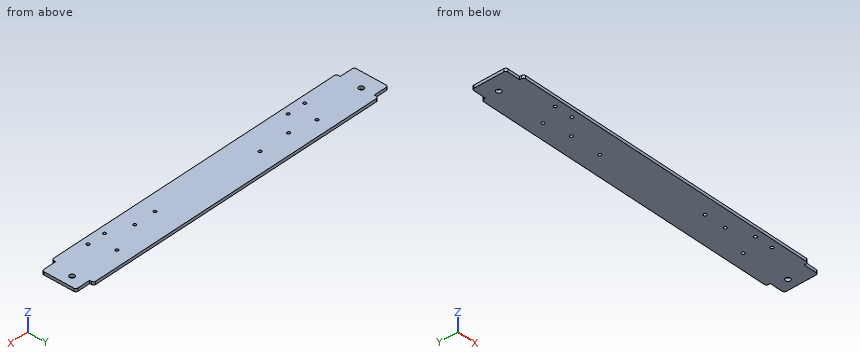
```python
from build123d import *

# Parameters (mm, degrees)
CROQUIS1_W                                 = 340
CROQUIS1_H                                 = 42
CROQUIS1_R                                 = 1.5
CROQUIS1_R_2                               = 2.5
SALIENTE_EXTRUIR1_DEPTH                    = 3
CROQUIS2_W                                 = 15
CROQUIS2_H                                 = 4
CORTAR_EXTRUIR2_DEPTH                      = 172.31841699
SIMETR_A4_AT_THE_SECOND_PLANE_COPY_1_SKE_W = 15
SIMETR_A4_AT_THE_SECOND_PLANE_COPY_1_SKE_H = 4
SIMETR_A4_AT_THE_SECOND_PLANE_COPY_1_DEPTH = 172.31841699
REDONDEO1_R                                = 2


with BuildPart() as part:
    # Croquis1 → Saliente-Extruir1 (new body)
    with BuildSketch(Plane.XY):
        Rectangle(CROQUIS1_W, CROQUIS1_H)
        with Locations((-47, 2)):
            Circle(CROQUIS1_R, mode=Mode.SUBTRACT)
        with Locations((-78, 2)):
            Circle(CROQUIS1_R, mode=Mode.SUBTRACT)
        with Locations((-104, 6.5)):
            Circle(CROQUIS1_R, mode=Mode.SUBTRACT)
        with Locations((-113, -14)):
            Circle(CROQUIS1_R, mode=Mode.SUBTRACT)
        with Locations((-95, -14)):
            Circle(CROQUIS1_R, mode=Mode.SUBTRACT)
        with Locations((-155, 4)):
            Circle(CROQUIS1_R_2, mode=Mode.SUBTRACT)
        with Locations((160, 4)):
            Circle(CROQUIS1_R_2, mode=Mode.SUBTRACT)
        with Locations((114, 6.5)):
            Circle(CROQUIS1_R, mode=Mode.SUBTRACT)
        with Locations((105, -14)):
            Circle(CROQUIS1_R, mode=Mode.SUBTRACT)
        with Locations((123, -14)):
            Circle(CROQUIS1_R, mode=Mode.SUBTRACT)
        with Locations((82, -5)):
            Circle(CROQUIS1_R, mode=Mode.SUBTRACT)
        with Locations((60, -5)):
            Circle(CROQUIS1_R, mode=Mode.SUBTRACT)
    extrude(amount=SALIENTE_EXTRUIR1_DEPTH)

    # Croquis2 → Cortar-Extruir2 (cut, through all)
    with BuildSketch(Plane.XY.offset(3)):
        with Locations((-162.5, -19)):
            Rectangle(CROQUIS2_W, CROQUIS2_H)
    cortar_extruir2 = extrude(amount=-CORTAR_EXTRUIR2_DEPTH, mode=Mode.SUBTRACT)

    # Simetría4: Cortar-Extruir2 across plane
    add(cortar_extruir2.mirror(Plane(origin=(0, 0, 0), x_dir=(0, 0, 1), z_dir=(1, 0, 0))), mode=Mode.SUBTRACT)

    # Simetría4 at the second plane: Cortar-Extruir2 across plane
    add(cortar_extruir2.mirror(Plane.ZX), mode=Mode.SUBTRACT)

    # Simetría4 at the second plane copy 1 ske → Simetría4 at the second plane copy 1 (cut, through all)
    with BuildSketch(Plane(origin=(0, 0, 3), x_dir=(-1, 0, 0), z_dir=(0, 0, 1))):
        with Locations((-162.5, -19)):
            Rectangle(SIMETR_A4_AT_THE_SECOND_PLANE_COPY_1_SKE_W, SIMETR_A4_AT_THE_SECOND_PLANE_COPY_1_SKE_H)
    extrude(amount=-SIMETR_A4_AT_THE_SECOND_PLANE_COPY_1_DEPTH, mode=Mode.SUBTRACT)

    # Redondeo1
    redondeo1_edges = [part.edges().sort_by_distance(p)[0] for p in [
        (155, -21, 1.5),
        (170, 17, 1.5),
        (155, 21, 1.5),
        (-170, -17, 1.5),
        (-155, -21, 1.5),
        (-170, 17, 1.5),
        (-155, 21, 1.5),
        (170, -17, 1.5),
    ]]
    fillet(redondeo1_edges, radius=REDONDEO1_R)


solid = part.part
```
Input: part model. Units: mm. Frame: model coordinates. Round coordinates to 2 decimals unless told otherwise and drop trailing zeros. Answer in a Markdown table with one row per item. Add a question column.
1. Section A-A (z = 1.25). Give the number of separate pieces and of enclosed holes in the cut face, and give its area (3 significant figures).
2. Ray query, probe 1 along Y at (x, z) = (160, 1.7); probe 2 along Y at (x, z) = (-113, 1.05); probe 3 along X at (y, z) = (2.5, 0.2). Return the intervals inside material, ascending.
3. Contact query for flat-ended pins moving along their axis: pin 1 (6 mm diameter, centred on x = 160, y = 4, fed in from -Z); pin 2 (1.6 mm diameter, centred on y = -18.5, z = 1, fed in from +X); pin 3 (0.6 mm diameter, centred on y = -18.5, z = 1.5, fed in from -X). Output: stop coordinate, or through.
Values follow:
| question | item | result |
|---|---|---|
| 1 | separate pieces | 1 |
| 1 | enclosed holes | 12 |
| 1 | area | 13,900 mm^2 |
| 2 | probe 1 | -17 to 1.5, 6.5 to 17 |
| 2 | probe 2 | -21 to -15.5, -12.5 to 21 |
| 2 | probe 3 | -170 to -157, -153 to -79.41, -76.59 to -48.41, -45.59 to 158, 162 to 170 |
| 3 | pin 1 | z = 0 |
| 3 | pin 2 | x = 155 |
| 3 | pin 3 | x = -155 |
